from build123d import *

# Parameters (mm, degrees)
SKETCH1_W                                           = 22
SKETCH1_H                                           = 170
BOSS_EXTRUDE1_DEPTH                                 = 14.5
SKETCH2_W                                           = 21
SKETCH2_H                                           = 79
CUT_EXTRUDE1_DEPTH                                  = 89.990167996
FILLET3_R                                           = 25
FILLET1_R                                           = 5
FILLET2_R                                           = 2
FILLET4_R                                           = 8
TAPPED_HOLE_FOR_M5X0_8_HELICOIL1_D                  = 5.2
CBORE_FOR_M4_HEX_SOCKET_HEAD_CAP_SCREW1_D           = 4.5
CBORE_FOR_M4_HEX_SOCKET_HEAD_CAP_SCREW1_CBORE_D     = 8
CBORE_FOR_M4_HEX_SOCKET_HEAD_CAP_SCREW1_CBORE_DEPTH = 4.4
SKETCH9_R                                           = 2.05
CUT_EXTRUDE2_DEPTH                                  = 89.990167996


with BuildPart() as part:
    # Sketch1 → Boss-Extrude1 (new, symmetric)
    with BuildSketch(Plane.XY):
        Rectangle(SKETCH1_W, SKETCH1_H)
    extrude(amount=BOSS_EXTRUDE1_DEPTH, both=True)

    # Sketch2 → Cut-Extrude1 (cut, through all)
    with BuildSketch(Plane(origin=(11, 0, 0), x_dir=(0, 0, -1), z_dir=(1, 0, 0))):
        with Locations((4, 45.5)):
            Rectangle(SKETCH2_W, SKETCH2_H)
    cut_extrude1 = extrude(amount=-CUT_EXTRUDE1_DEPTH, mode=Mode.SUBTRACT)

    # Mirror1: Cut-Extrude1 across plane
    add(cut_extrude1.mirror(Plane.ZX), mode=Mode.SUBTRACT)

    # Fillet3
    # the kernel refuses this fillet: 25 mm, written as the material it adds along each edge
    with BuildSketch(Plane(origin=(11, 6, 6.5), x_dir=(0, 0, -1), z_dir=(-1, 0, 0))) as fillet3_piece_1:
        with BuildLine():
            CenterArc((25, -24.677925359), FILLET3_R, 99.206896221, 80.793103779)
            Line((0, -24.677925359), (-0.5, -24.677925359))
            Line((-0.5, -24.677925359), (-0.5, 0))
            Line((-0.5, 0), (0, 0.5))
            ThreePointArc((0, 0.5), (10.5, 0.5), (20.92, 0.493558507))
            Line((20.92, 0.493558507), (21, 0))
        make_face()
    extrude(amount=22)
    with BuildSketch(Plane(origin=(11, -6, 6.5), x_dir=(0, -1, 0), z_dir=(-1, 0, 0))) as fillet3_piece_2:
        with BuildLine():
            CenterArc((24.677925359, -25), FILLET3_R, 90, 80.793103779)
            Line((0, -21), (-0.493558507, -20.92))
            ThreePointArc((-0.493558507, -20.92), (-0.5, -10.5), (-0.5, 0))
            Line((-0.5, 0), (0, 0.5))
            Line((0, 0.5), (24.677925359, 0.5))
            Line((24.677925359, 0.5), (24.677925359, 0))
        make_face()
    extrude(amount=22)

    # Fillet1
    fillet1_edges = [part.edges().sort_by_distance(p)[0] for p in [
        (11, -85, 10.5),
        (-11, -85, 10.5),
        (-11, 85, 10.5),
        (11, 85, 10.5),
    ]]
    fillet(fillet1_edges, radius=FILLET1_R)

    # Fillet2
    fillet2_edges = [part.edges().sort_by_distance(p)[0] for p in [
        (11, 0, 14.5),
        (0, -85, 14.5),
        (0, 85, 14.5),
        (-11, 0, 14.5),
        (9.535533906, 83.535533906, 14.5),
        (-9.535533906, 83.535533906, 14.5),
        (-9.535533906, -83.535533906, 14.5),
        (9.535533906, -83.535533906, 14.5),
    ]]
    fillet(fillet2_edges, radius=FILLET2_R)

    # Fillet4
    # the kernel refuses this fillet: 8 mm, written as the material it takes off along each edge
    with BuildSketch(Plane(origin=(26.157317348, -6, -14.5), x_dir=(0, 1, 0), z_dir=(-1, 0, 0))) as fillet4_piece_1:
        with BuildLine():
            CenterArc((6.062926939, -8), FILLET4_R, 90, 68.676313737)
            ThreePointArc((-1.38940089, -5.090909091), (-0.559998083, -2.582217249), (0, 0))
            Line((0, 0), (6.062926939, 0))
        make_face()
    extrude(amount=52.314634697, mode=Mode.SUBTRACT)
    with BuildSketch(Plane(origin=(26.157317348, 6, -14.5), x_dir=(0, 0.2632886899666048, 0.96471709103533), z_dir=(-1, 0, 0))) as fillet4_piece_2:
        with BuildLine():
            CenterArc((6.121436637, -7.95531876), FILLET4_R, 96.058395021, 68.676313736)
            Line((-1.596300091, -5.84900924), (0, 0))
            ThreePointArc((0, 0), (2.638550275, -0.139628875), (5.277100549, 0))
        make_face()
    extrude(amount=52.314634697, mode=Mode.SUBTRACT)

    # Tapped Hole for M5x0.8 Helicoil1 (through all)
    with Locations(Plane.XY.offset(14.5)):
        with Locations((0, 75)):
            tapped_hole_for_m5x0_8_helicoil1 = Hole(TAPPED_HOLE_FOR_M5X0_8_HELICOIL1_D / 2)

    # Mirror2: Tapped Hole for M5x0.8 Helicoil1 across plane
    add(tapped_hole_for_m5x0_8_helicoil1.mirror(Plane.ZX), mode=Mode.SUBTRACT)

    # CBORE for M4 Hex Socket Head Cap Screw1 (through all)
    with Locations(Plane.XY.offset(14.5)):
        with Locations((0, -60.0028)):
            CounterBoreHole(CBORE_FOR_M4_HEX_SOCKET_HEAD_CAP_SCREW1_D / 2, CBORE_FOR_M4_HEX_SOCKET_HEAD_CAP_SCREW1_CBORE_D / 2, CBORE_FOR_M4_HEX_SOCKET_HEAD_CAP_SCREW1_CBORE_DEPTH)

    # Sketch9 → Cut-Extrude2 (cut, through all)
    with BuildSketch(Plane(origin=(11, 0, 0), x_dir=(0, 0, -1), z_dir=(1, 0, 0))):
        with Locations((7.517, 0)):
            Circle(SKETCH9_R)
    extrude(amount=-CUT_EXTRUDE2_DEPTH, mode=Mode.SUBTRACT)


solid = part.part
Build history of the part. All positions in model axes, mm. A direction names the side the tool comes from. Round coordinates to 2 decimals unless told otherwise and drop trailing zeros. Loops run counter-clockwise (first coordinate to the right, second up) from the corner with the lowest first, then second, coordinate; pieces in that order, holes last. Notation, with made-up numbers: (39.5, -17.5) -> (77.5, -17.5) arc R18 ccw to (77.5, -4.5) -> close; hole circle Ø5 at (20.25, -35). An arc over 180 degrees is marked (long way). Use CSV: the item, a comma, the result in double quotes. Start each with the question number.
Q1. Which spindle directions (+Z, -Z, +X, -X, +Y, -Y) get a long thin tool onto all of the face, cutting with end or side? Do faces 1 (the face through (11, 0, 6)), 2 (the face through (0, -57, 6.5)), 3 (the face through (0, 57, 6.5)). Say none if no direction does.
Q2. Mould opens along Y. For faces 4 (the face through (0, -85, 10)), 5 (the face through (-10, 83, 9)), 6 (the face through (-0.521, -56.037, 12.331)) say: +Y half, -Y half, draft (parallel to the pull), parting line (faces both ways), or undercut.
Q3. Saw through at B-B on y = 75. Give the cut face in (x, z), and give its area (3 significant figures).
Q4. Saw through at C-C on y = 19. Give the cut face in (x, z), and give its area (3 significant figures).
Q5. Flat gauge pins, fed straight in: pin 1 Ø12 at (y, z) = (29, 1.5) entering from -X; pin 2 Ø6.5 at (x, y) = (0, -60) entering from -Z; pin 3 Ø1 at (x, z) = (-7.5, -9.5) entering from +Y; pin 4 Ø4 at (x, z) = (2, -5.5) entering from -Y. Where does each tip first touch, or does it go through?
Q6. Saw through at A-A on x = 0. Give the cut face in (y, z).
Q7. Drill centre lines: L1, parallel to Y at x = 0, z = 12; L2, parallel to Y at x = 0, z = 8.35; L3, parallel to Z at x = 8.25, y = -61. Where is each one in solid material? Low to high.
Solutions:
1,face 1,"+Z, -Z, +X, +Y, -Y"
1,face 2,"-Z, +X, -X, -Y"
1,face 3,"-Z, +X, -X, +Y"
2,face 4,"-Y half"
2,face 5,"+Y half"
2,face 6,"undercut"
3,outline,"(-11, 6.5) -> (-2.6, 6.5) -> (-2.6, 14.5) -> (-9, 14.5) arc R2 ccw to (-11, 12.5) -> close; (2.6, 6.5) -> (11, 6.5) -> (11, 12.5) arc R2 ccw to (9, 14.5) -> (2.6, 14.5) -> close"
3,area,"133 mm^2"
4,outline,"(-11, 3.6) -> (11, 3.6) -> (11, 12.5) arc R2 ccw to (9, 14.5) -> (-9, 14.5) arc R2 ccw to (-11, 12.5) -> close"
4,area,"238 mm^2"
5,pin 1,"stops at x = -11"
5,pin 2,"stops at z = 6.5"
5,pin 3,"stops at y = 7.55"
5,pin 4,"stops at y = -10.68"
6,outline,"(-85, 6.5) -> (-77.6, 6.5) -> (-77.6, 14.5) -> (-83, 14.5) arc R2 ccw to (-85, 12.5) -> close; (-72.4, 6.5) -> (-62.25, 6.5) -> (-62.25, 10.1) -> (-64, 10.1) -> (-64, 14.5) -> (-72.4, 14.5) -> close; (-57.75, 6.5) -> (-30.68, 6.5) arc R25 cw to (-7.39, -9.41) arc R8 ccw to (0, -14.5) arc R8 ccw to (7.39, -9.41) arc R25 cw to (30.68, 6.5) -> (72.4, 6.5) -> (72.4, 14.5) -> (-56, 14.5) -> (-56, 10.1) -> (-57.75, 10.1) -> close; (77.6, 6.5) -> (85, 6.5) -> (85, 12.5) arc R2 ccw to (83, 14.5) -> (77.6, 14.5) -> close; hole circle Ø4.1 at (0, -7.52)"
7,L1,"y = -85 to -77.6, -72.4 to -64, -56 to 72.4, 77.6 to 85"
7,L2,"y = -85 to -77.6, -72.4 to -62.25, -57.75 to 72.4, 77.6 to 85"
7,L3,"z = 6.5 to 14.5"
